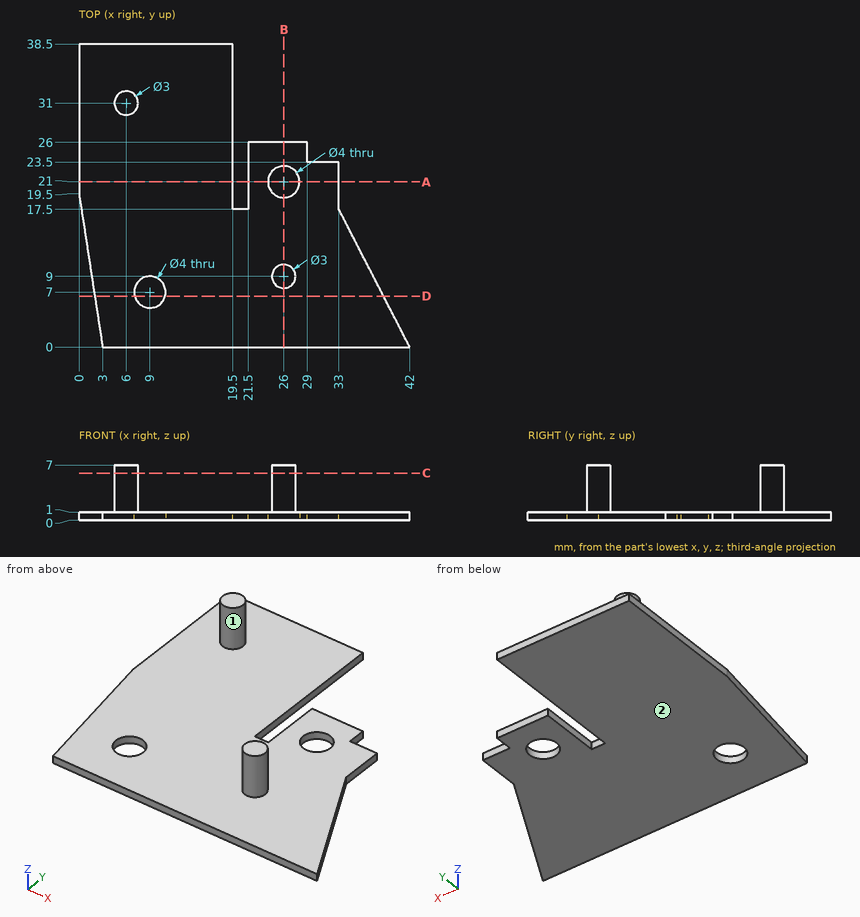
Source: three-view drawing plus pictorial views. Frame: mm from the lowest corner of the part. A direction names the side the tool comes from. Give positions to 0.01 mm unless a question says otherwise; leave off trailing zeros. Order: outer loops, then holes, each group sorted by start corner. A loop starts at its lowest first (then second) coordinate and runs counter-clockwise, first axis right, second up. Notation, with made-up numbers: M 22.5,51.5 L 61.5,51.5 A25 cw 61.5,73.5 Z; hole C 82.5,61 d4. An arc over 180 degrees is marked long. Return JSON: item names as keys, results as strings.
1) Contact query for flat-ended pins moving along their axis: pin 1 (4.5 mm diameter, centred on x = 26, y = 21, fed in from +Z); pin 2 (0.8 mm diameter, centred on x = 31, z = 0.5, fed in from +Y); pin 3 (3.5 mm diameter, centred on x = 9, y = 7, fed in from +Z); pin 4 (0.5 mm diameter, centred on y = 24.5, z = 0.5, fed in from +X). Output: stop coordinate, or through.
Taken from the geometry:
{"pin 1": "stops at z = 1", "pin 2": "stops at y = 23.5", "pin 3": "passes through", "pin 4": "stops at x = 29"}
2) Line query: L1, parallel to Y at x = 26, z = 0.35; L2, parallel to Y at x = 9, z = 0.8; L3, parallel to Z at x = 13.5, y = 15. Output: solid intervals per line, ascending. Write a range as [from, to].
Taken from the geometry:
{"L1": "y = [0, 19], [23, 26]", "L2": "y = [0, 5], [9, 38.5]", "L3": "z = [0, 1]"}
3) Section query A-A on y = 21. Output: boundary loops of the cut face in (x, z), and give its area (3 significant figures).
Taken from the geometry:
{"outline": "M 0,0 L 19.5,0 L 19.5,1 L 0,1 Z; M 21.5,0 L 24,0 L 24,1 L 21.5,1 Z; M 28,0 L 33,0 L 33,1 L 28,1 Z", "area": "27.0 mm2"}
4) Section query D-D on y = 6.5. Output: boundary loops of the cut face in (x, z).
Taken from the geometry:
{"outline": "M 2,0 L 7.06,0 L 7.06,1 L 2,1 Z; M 10.94,0 L 38.66,0 L 38.66,1 L 10.94,1 Z"}
5) Section query C-C on z = 6. Output: boundary loops of the cut face in (x, y), and give its area (3 significant figures).
Taken from the geometry:
{"outline": "C 6,31 d3; C 26,9 d3", "area": "14.1 mm2"}
6) Access query for the marked faces 1 and 2. Directions: +Z, -Z, +X, -X, +Y, -Y. A direction counts if a zero-diameter tool reaches every point of the face in a straight line with its end or side. Return the directions, or none.
Taken from the geometry:
{"face 1": "+Z", "face 2": "-Z, +X, -X, +Y, -Y"}
7) Section query B-B on x = 26. Output: boundary loops of the cut face in (y, z).
Taken from the geometry:
{"outline": "M 0,0 L 19,0 L 19,1 L 10.5,1 L 10.5,7 L 7.5,7 L 7.5,1 L 0,1 Z; M 23,0 L 26,0 L 26,1 L 23,1 Z"}
